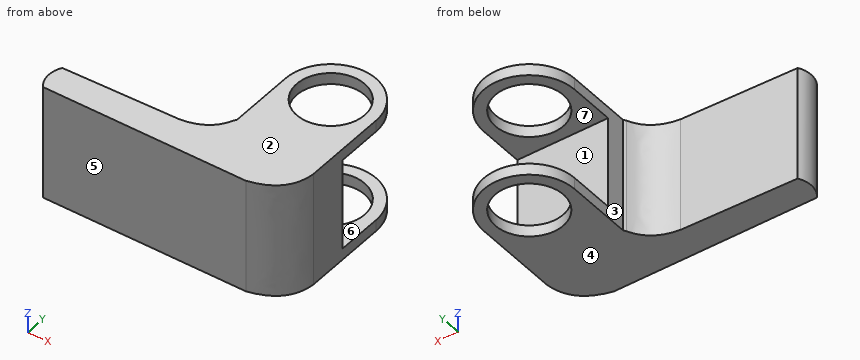
```python
from build123d import *

# Parameters (mm, degrees)
SKETCH1_R           = 8.9
BOSS_EXTRUDE1_DEPTH = 30
SKETCH2_W           = 24
SKETCH2_H           = 23.8
CUT_EXTRUDE1_DEPTH  = 23.8


with BuildPart() as part:
    # Sketch1 → Boss-Extrude1 (new body)
    with BuildSketch(Plane.XY):
        with BuildLine():
            ThreePointArc((11.9, 0), (0, 11.9), (-11.9, 0))
            Line((-11.9, 0), (-11.9, -16.75270202))
            Line((-11.9, -16.75270202), (-11.9, -17.254561811))
            Line((-11.9, -17.254561811), (-12.301407367, -17.836587713))
            add(Edge.make_bspline(
                [(-21.764559413, -24.28445135), (-14.705345203, -23.52602921), (-12.301407367, -17.836587713)],
                knots=[0, 0, 0, 0.916072404, 0.916072404, 0.916072404], degree=2))
            Line((-21.764559413, -24.28445135), (-51.930587301, -25.04963318))
            ThreePointArc((-51.930587301, -25.04963318), (-52.886196001, -28.917406192), (-51.420694634, -32.62215474))
            Line((-51.420694634, -32.62215474), (1.732240064, -32.62215474))
            add(Edge.make_bspline(
                [(1.732240064, -32.62215474), (11.248165951, -30.665230595), (11.9, -22.221272353)],
                knots=[0, 0, 0, 1, 1, 1], degree=2))
            Line((11.9, -22.221272353), (11.9, 0))
        make_face()
        Circle(SKETCH1_R, mode=Mode.SUBTRACT)
    extrude(amount=BOSS_EXTRUDE1_DEPTH)

    # Sketch2 → Cut-Extrude1 (cut)
    with BuildSketch(Plane.ZY.offset(11.9)):
        with Locations((15, 0)):
            Rectangle(SKETCH2_W, SKETCH2_H)
    extrude(amount=-CUT_EXTRUDE1_DEPTH, mode=Mode.SUBTRACT)


solid = part.part
```
Here's how the part is built. I have some questions about the finished solid (model axes, mm). Face numbers are marked on the shaded views. A direction names the side the tool comes from. Coordinates: 2 decimals unless noted, no trailing zeros. Loops run counter-clockwise (first coordinate to the right, second up) from the corner with the lowest first, then second, coordinate; pieces in that order, holes last. Notation, with made-up numbers: (-25.75, -33) - (-14.75, -33) arc R15 cw to (-14.75, -18) - close; hole circle Ø5 at (29.5, 54.25). An arc over 180 degrees is marked (long way). Return JSON: item names as keys, results as strings. Group by question number.
Item 1: On a 3-axis mill with a long thin cutter (end or side, diameter ignored), from which of +Z, -Z, +X, -X, +Y, -Y can I reach the whole of each face in a straight line? I mean the marked faces 1, 2 and 3. Say none if no direction works.
Item 2: If we section it at B-B on y = -10: Write out the boundary of the cut face in (x, z).
Item 3: If we section it at C-C on y = -1.5: Write out the boundary of the cut face in (x, z), and give its area (3 significant figures).
Item 4: If we section it at D-D on y = 6: Write out the boundary of the cut face in (x, z), and give its area (3 significant figures).
Item 5: We'd pull the mould along Z, two halves only. Please class the marked faces 4, 5, 6 and 7: +Z half, -Z half, draft (parallel to the pull), parting line (faces both ways), or undercut.
Item 6: If we section it at A-A on x = 0: Write out the boundary of the cut face in (y, z), and give its area (3 significant figures).
Item 7: I need wall thicknesses on line 1 (Y direction, x = 0, z = 1); line 2 (Z direction, x = 8.5, y = -9.5); line 3 (Y direction, x = -7, z = 7). Which ranges of each line are inside material? Lowest first, please. Write a range as from..to.
Item 8: Will these pins go through, and if not, where does the flat tip stop? P1, Ø2, axis at x = -31, z = 17.5, coming from the +Y side; P2, Ø10, axis at x = -10, z = 14, coming from the +Y side; P3, Ø2, axis at x = -26, z = 13, coming from the +Y side; P4, Ø12, axis at x = -5.5, y = 5, coming from the -Z side.
Calculated:
{
 "1": {"face 1": "+X, -X, +Y", "face 2": "+Z, +X, -X, +Y, -Y", "face 3": "+Z, -Z, -X, +Y"},
 "2": {"outline": "(-11.9, 0) - (11.9, 0) - (11.9, 3) - (-11.9, 3) - close; (-11.9, 27) - (11.9, 27) - (11.9, 30) - (-11.9, 30) - close"},
 "3": {"outline": "(-11.9, 0) - (-8.77, 0) - (-8.77, 3) - (-11.9, 3) - close; (-11.9, 27) - (-8.77, 27) - (-8.77, 30) - (-11.9, 30) - close; (8.77, 0) - (11.9, 0) - (11.9, 3) - (8.77, 3) - close; (8.77, 27) - (11.9, 27) - (11.9, 30) - (8.77, 30) - close", "area": "37.5 mm^2"},
 "4": {"outline": "(-10.28, 0) - (-6.57, 0) - (-6.57, 3) - (-10.28, 3) - close; (-10.28, 27) - (-6.57, 27) - (-6.57, 30) - (-10.28, 30) - close; (6.57, 0) - (10.28, 0) - (10.28, 3) - (6.57, 3) - close; (6.57, 27) - (10.28, 27) - (10.28, 30) - (6.57, 30) - close", "area": "44.4 mm^2"},
 "5": {"face 4": "-Z half", "face 5": "draft", "face 6": "undercut", "face 7": "undercut"},
 "6": {"outline": "(-32.62, 0) - (-8.9, 0) - (-8.9, 3) - (-11.9, 3) - (-11.9, 27) - (-8.9, 27) - (-8.9, 30) - (-32.62, 30) - close; (8.9, 0) - (11.9, 0) - (11.9, 3) - (8.9, 3) - close; (8.9, 27) - (11.9, 27) - (11.9, 30) - (8.9, 30) - close", "area": "658 mm^2"},
 "7": {"line 1": "y = -32.62..-8.9, 8.9..11.9", "line 2": "z = 0..3, 27..30", "line 3": "y = -32.62..-11.9"},
 "8": {"P1": "stops at y = -24.49", "P2": "stops at y = -11.9", "P3": "stops at y = -24.37", "P4": "stops at z = 0"}
}
